Design review of the part shown in the three views and the two pictorial views. Dimensions are in mm from the part's minimum x, y and z. Coordinates: 2 decimals unless noted, no trailing zeros. Write each loop counter-clockwise with the first axis right and the second up, starting at its lowest first coordinate (ties: lowest second). Pieces come first, ordered by that corner, then holes. Notation, with made-up numbers: M 44.5,69 L 100.5,69 A19 cw 100.5,88 Z; hole C 50,-38.75 d10. An arc over 180 degrees is marked long. One line per question, with ' | ' between items.
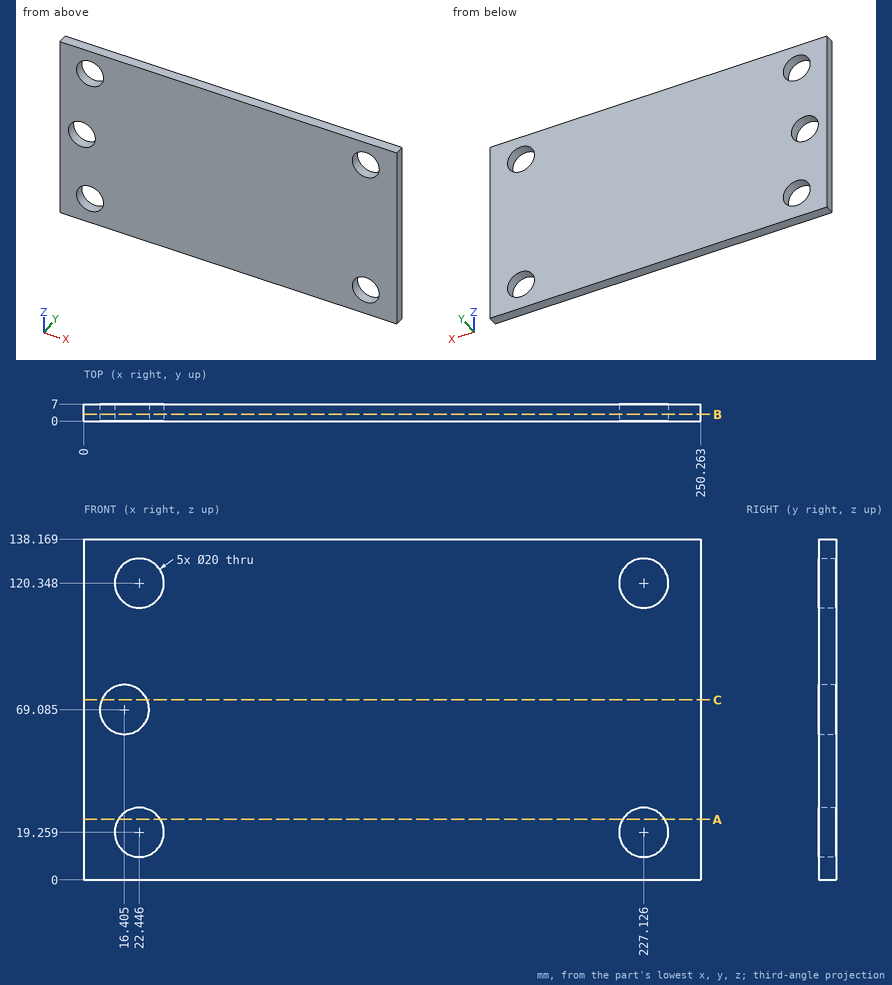
1. Take a section at A-A on z = 24.5. State the section outline as (x, y) points, plus the area to 3 significant figures.
Computed values:
outline: M 0,0 L 13.93,0 L 13.93,7 L 0,7 Z; M 30.96,0 L 218.61,0 L 218.61,7 L 30.96,7 Z; M 235.64,0 L 250.26,0 L 250.26,7 L 235.64,7 Z | area: 1,510 mm2
2. Take a section at B-B on y = 2.75. State the section outline as (x, z) points (1 decimal).
Computed values:
outline: M 0,0 L 250.3,0 L 250.3,138.2 L 0,138.2 Z; hole C 16.4,69.1 d20; hole C 22.4,19.3 d20; hole C 22.4,120.3 d20; hole C 227.1,19.3 d20; hole C 227.1,120.3 d20
3. Take a section at C-C on z = 73. State the section outline as (x, y) points, plus the area to 3 significant figures.
Computed values:
outline: M 0,0 L 7.2,0 L 7.2,7 L 0,7 Z; M 25.61,0 L 250.26,0 L 250.26,7 L 25.61,7 Z | area: 1,620 mm2
4. For line 1 along X through (y, z) = (2.75, 19.5); line 2 along X through (y, z) = (1, 119.5); line 3 along X through (y, z) = (1, 71.5), list the stretches that pass through material, from the lowest coordinate up.
Computed values:
line 1: x = 0 to 12.45, 32.44 to 217.13, 237.12 to 250.26 | line 2: x = 0 to 12.48, 32.41 to 217.16, 237.09 to 250.26 | line 3: x = 0 to 6.7, 26.11 to 250.26
